```python
from build123d import *

# Parameters (mm, degrees)
F0_R     = 205.633552
F0_R_2   = 164.498916
F1_DEPTH = 812.8
F2_R     = 256.008215
F3_DEPTH = 50.8
F4_R     = 261.306148
F4_R_2   = 166.325604
F5_DEPTH = 38.1
F7_D     = 25.4
F7_DEPTH = 50.8


with BuildPart() as f1:
    # F0 (on Top) → F1 (new body)
    with BuildSketch(Plane.XY):
        Circle(F0_R)
        Circle(F0_R_2, mode=Mode.SUBTRACT)
    extrude(amount=-F1_DEPTH)

    # F2 (on face) → F3 (join)
    with BuildSketch(Plane(origin=(0, 0, -812.8), x_dir=(1, 0, 0), z_dir=(0, 0, -1))):
        Circle(F2_R)
    extrude(amount=F3_DEPTH)

    # F4 (on face) → F5 (join)
    with BuildSketch(Plane.XY):
        Circle(F4_R)
        Circle(F4_R_2, mode=Mode.SUBTRACT)
    extrude(amount=F5_DEPTH)

    # F7
    with Locations(Plane.XY.offset(38.1)):
        with Locations((87.061769, 215.107856), (161.676934, 166.468347), (212.168418, 93.998425), (232.058487, 0), (216.818106, -82.710644), (170.387229, -157.54153), (90.523878, -213.673978), (0, -232.058487), (-91.290017, -213.347778), (-165.596627, -162.569673), (-214.243309, -89.168077), (-232.058487, 0), (-212.893799, 92.34377), (-165.596627, 162.569673), (-87.061769, 215.107856), (0, 232.058487)):
            Hole(F7_D / 2, depth=F7_DEPTH)


solid = f1.part
```
Build history of the part. All positions in model axes, mm. A direction names the side the tool comes from. Round coordinates to 2 decimals unless told otherwise and drop trailing zeros. Write each loop counter-clockwise with the first axis right and the second up, starting at its lowest first coordinate (ties: lowest second). Pieces come first, ordered by that corner, then holes.
1) Mould opens along X. For faces 1 (the cylindrical face through (-203.159, 155.777, -837.844)), 2 (the flat face through (171, 4, 38.1)), 3 (the cylindrical face through (2.75, 219.66, 18.78)) say: +X half, -X half, draft (parallel to the pull), parting line (faces both ways), or undercut.
2) 3-axis set-ups, long thin cutter, end or side, ignore diameter. For faces 4 (the cylindrical face through (-56.65, -255.09, 18.78)), 5 (the cylindrical face through (-205.435, 9.041, -400.71)), 6 (the cylindrical face through (155.82, 155.2, 18.78)): which of +Z, -Z, +X, -X, +Y, -Y reach the whole face in a straight line?
3) Drill centre lines: probe 1 along Y at (x, z) = (0, 22); probe 2 along Z at (x, y) = (-53, -148); probe 3 along X at (y, z) = (-102.5, -478.5). Where is each one in solid material? Low to high.
4) Pin check, flat tips, straight feed: pin 1 (10 mm diameter, centred on y = 40.5, z = -201.5, fed in from +X); pin 2 (6 mm diameter, centred on x = -71, z = -753.5, fed in from -Y); pin 3 (12 mm diameter, centred on x = 50, z = -119.5, fed in from +Y). Stop position of each tip, or through.
5) Band-saw the part on D-D, the plane x = 126. List the corners of the cut face in (y, z), and give its area (3 significant figures).
6) Band-saw the part on A-A, the plane x = 0. List the corners of the cut face in (y, z).
7) Band-saw the part on C-C, the plane z = -442. List the corners of the cut face in (x, y), and give its area (3 significant figures).
Ans:
1. face 1: parting line
1. face 2: draft
1. face 3: undercut
2. face 4: +Z, -Z
2. face 5: none
2. face 6: +Z
3. probe 1: y = -261.31 to -244.76, -219.36 to -166.33, 166.33 to 219.36, 244.76 to 261.31
3. probe 2: z = -863.6 to -812.8
3. probe 3: x = -178.27 to -128.66, 128.66 to 178.27
4. pin 1: stops at x = 202.55
4. pin 2: stops at y = -194.06
4. pin 3: stops at y = 200.87
5. outline: (-228.92, 0) - (-162.51, 0) - (-162.51, -812.8) - (-222.85, -812.8) - (-222.85, -863.6) - (222.85, -863.6) - (222.85, -812.8) - (162.51, -812.8) - (162.51, 0) - (228.92, 0) - (228.92, 38.1) - (108.57, 38.1) - (108.57, 0) - (105.75, 0) - (105.75, -812.8) - (-105.75, -812.8) - (-105.75, 0) - (-108.57, 0) - (-108.57, 38.1) - (-228.92, 38.1) - close
5. area: 124,000 mm2
6. outline: (-261.31, 0) - (-244.76, 0) - (-244.76, 38.1) - (-261.31, 38.1) - close; (-256.01, -863.6) - (256.01, -863.6) - (256.01, -812.8) - (205.63, -812.8) - (205.63, 0) - (219.36, 0) - (219.36, 38.1) - (166.33, 38.1) - (166.33, 0) - (164.5, 0) - (164.5, -812.8) - (-164.5, -812.8) - (-164.5, 0) - (-166.33, 0) - (-166.33, 38.1) - (-219.36, 38.1) - (-219.36, 0) - (-205.63, 0) - (-205.63, -812.8) - (-256.01, -812.8) - close; (244.76, 0) - (261.31, 0) - (261.31, 38.1) - (244.76, 38.1) - close
7. outline: circle Ø411.27 at (0, 0); hole circle Ø329 at (0, 0)
7. area: 47,800 mm2
